Check sheet for the modelled part. Datum: model origin and axes. Units: mm. A direction names the side the tool comes from. Round coordinates to 2 decimals unless told otherwise and drop trailing zeros. Write each loop counter-clockwise with the first axis right and the second up, starting at its lowest first coordinate (ties: lowest second). Pieces come first, ordered by that corner, then holes. Notation, with made-up numbers: M 14.5,61 L 59.5,61 A22 cw 59.5,74 Z; hole C -35.5,-20.75 d8. An arc over 180 degrees is marked long. One line per item, written item: value.
Autodesk Inventor part; units mm, degrees
ref_plane "YZ Plane" through (0, 0, 0) normal (1, 0, 0) x (0, 1, 0)
ref_plane "XZ Plane" through (0, 0, 0) normal (0, 1, 0) x (-1, 0, 0)
ref_plane "XY Plane" through (0, 0, 0) normal (0, 0, 1) x (1, 0, 0)
sketch "Sketch1" plane through (0, 0, 0) normal (0, 0, 1) x (1, 0, 0)
  circle A0 centre (0, 0) radius 2.75
  dimension "d0" = 5.5
extrude "Extrusion1" add sketch "Sketch1" against normal blind 3
sketch "Sketch2" plane through (0, 0, 0) normal (0, 0, 1) x (1, 0, 0)
  circle A0 centre (0, 0) radius 1.5
  dimension "d3" = 3
extrude "Extrusion2" add sketch "Sketch2" along normal blind 5
chamfer "Chamfer1" distance 0.3 angle 45 2 edges at (-2.75, 0, -3) (-1.5, 0, 5)
sketch "Sketch3" plane through (0, 0, -3) normal (0, 0, -1) x (-1, 0, 0)
  line L0 (-0.7217, -1.25) -> (-1.4434, 0)
  line L1 (-1.4434, 0) -> (-0.7217, 1.25)
  line L2 (-0.7217, 1.25) -> (0.7217, 1.25)
  line L3 (0.7217, 1.25) -> (1.4434, 0)
  line L4 (1.4434, 0) -> (0.7217, -1.25)
  line L5 (0.7217, -1.25) -> (-0.7217, -1.25)
  point P0 (0, 0)
  point P1 (0, 0)
  dimension "d9" = 2.5
extrude "Extrusion3" cut sketch "Sketch3" against normal blind 2
properties part number "socket_head_cap_screw_M3x5"
Q1. Sectioned sample at A-A on z = -2. Enter the section's corners in (x, y).
Completed:
outline: C 0,0 d5.5; hole M -1.44,0 L -0.72,-1.25 L 0.72,-1.25 L 1.44,0 L 0.72,1.25 L -0.72,1.25 Z
Q2. Sectioned sample at C-C on z = 3.5. Enter the section's corners in (x, y), and give its area (3 significant figures).
Completed:
outline: C 0,0 d3
area: 7.07 mm^2
Q3. Scan lines: line 1 (Z direction, x = 1.15, y = 1.7); line 2 (Y direction, x = 0, z = 2.75); line 3 (Z direction, x = -0.1, y = -0.5). Record each from-to range of solid material in increasing order. Write a range as [from, to].
Completed:
line 1: [-3, 0]
line 2: [-1.5, 1.5]
line 3: [-1, 5]
Q4. Sectioned sample at B-B on x = 0. Enter the section's corners in (y, z), and give its area (3 significant figures).
Completed:
outline: M -2.75,-2.7 L -2.45,-3 L -1.25,-3 L -1.25,-1 L 1.25,-1 L 1.25,-3 L 2.45,-3 L 2.75,-2.7 L 2.75,0 L 1.5,0 L 1.5,4.7 L 1.2,5 L -1.2,5 L -1.5,4.7 L -1.5,0 L -2.75,0 Z
area: 26.3 mm^2
Q5. Draft check along Y on faces 4 (the cylindrical face through (-0.596, -2.685, -1.331)), 5 (the flat face through (-1.088, -0.616, -2.014)), 6 (the flat face through (0, 0, -1)), 7 (the flat face through (1.2, -1.2, 0)). Enter one of: pulls with the +Y half, pulls with the -Y half, needs draft (parallel to the pull), parting line crosses it, or undercut.
Completed:
face 4: parting line crosses it
face 5: undercut
face 6: undercut
face 7: needs draft
Q6. Access from +Z, -Z, +X, -X, +Y, -Y to the whole of each face (thin tool, end or side, straight path). Record for faces 1 (the cylindrical face through (-1.5, -0.07, 2.32)), 2 (the flat face through (1.1, -1.1, -3)), 3 (the flat face through (1.088, 0.616, -2.014)).
Completed:
face 1: +Z
face 2: -Z, +X, -X, +Y, -Y
face 3: -Z
Q7. Depth check by flat-ended pin: P1, Ø1.5, axis at x = 2, y = -0.5, coming from the +Z side; P2, Ø0.8, axis at x = 0.5, y = -0.5, coming from the -Z side; P3, Ø3, axis at x = 1, z = 3.5, coming from the -Y side. Enter the tip coordinate at first touch or a pass-through.
Completed:
P1: z = 4.89
P2: z = -1
P3: y = -1.5
